from build123d import *

# Parameters (mm, degrees)
F0_W      = 44
F0_H      = 60
F1_DEPTH  = 20
F2_W      = 2.5
F2_H      = 17
F3_DEPTH  = 20
F4_T      = -1.5
F5_W      = 5
F5_H      = 15
F6_DEPTH  = 2
F7_W      = 14
F7_H      = 2
F7_H_2    = 14
F8_DEPTH  = 7
F10_DEPTH = 14
F11_W     = 4
F11_H     = 4
F12_DEPTH = 18.5
F13_R     = 1.05
F14_DEPTH = 15
F15_W     = 7.7
F15_H     = 4.2
F16_DEPTH = 1.5
F17_W     = 2
F17_H     = 43.7
F17_H_2   = 39.7
F18_DEPTH = 5
F19_W     = 3
F19_H     = 10
F20_DEPTH = 12
F21_W     = 6
F21_H     = 2
F22_DEPTH = 10


# Not quite as in the source:
# - a pattern or mirror of a feature is missing from the dataset's text; its kind, count and spacing are read off the source's solid


with BuildPart() as f1:
    # F0 (on Top) → F1 (new body)
    with BuildSketch(Plane.XY):
        Rectangle(F0_W, F0_H)
    extrude(amount=F1_DEPTH)

    # F2 (on face) → F3 (cut)
    with BuildSketch(Plane.XY.offset(20)):
        with Locations((20.75, 0)):
            Rectangle(F2_W, F2_H)
        with Locations((-20.75, 0)):
            Rectangle(F2_W, F2_H)
    extrude(amount=-F3_DEPTH, mode=Mode.SUBTRACT)

    # F4
    f4_openings = [f1.faces().sort_by_distance(p)[0] for p in [
        (0, 0, 20),
    ]]
    offset(amount=F4_T, openings=f4_openings, kind=Kind.INTERSECTION)

    # F5 (on face) → F6 (cut)
    with BuildSketch(Plane(origin=(0, 0, 0), x_dir=(1, 0, 0), z_dir=(0, 0, -1))):
        with Locations((-16.5, -21)):
            Rectangle(F5_W, F5_H)
    extrude(amount=-F6_DEPTH, mode=Mode.SUBTRACT)

    # F7 (on face) → F8 (join)
    with BuildSketch(Plane.YZ.offset(19.5)):
        with Locations((0, 21)):
            Rectangle(F7_W, F7_H)
        with Locations((0, 13)):
            Rectangle(F7_W, F7_H_2)
    f8 = extrude(amount=F8_DEPTH)

    # F8_copies: F8 across plane
    add(f8.mirror(Plane(origin=(0, 0, 0), x_dir=(0, 0, -1), z_dir=(-1, 0, 0))))

    # F9 (on face) → F10 (cut)
    with BuildSketch(Plane.XZ.offset(7)):
        Polygon((23, 16.5), (19.5, 6), (26.5, 6), (26.5, 20), (22, 20), (22, 16.5), align=None)
    f10 = extrude(amount=-F10_DEPTH, mode=Mode.SUBTRACT)

    # F10_copies: F10 across plane
    add(f10.mirror(Plane(origin=(0, 0, 0), x_dir=(0, 0, -1), z_dir=(-1, 0, 0))), mode=Mode.SUBTRACT)

    # F11 (on face) → F12 (join, through all)
    with BuildSketch(Plane.XY.offset(1.5)):
        with Locations((18.5, 26.5)):
            Rectangle(F11_W, F11_H)
        with Locations((18.5, -26.5)):
            Rectangle(F11_W, F11_H)
        with Locations((-18.5, -26.5)):
            Rectangle(F11_W, F11_H)
        with Locations((-10, 26.5)):
            Rectangle(F11_W, F11_H)
    extrude(amount=F12_DEPTH)

    # F13 (on face) → F14 (cut)
    with BuildSketch(Plane.XY.offset(20)):
        with Locations((-10, 26.5)):
            Circle(F13_R)
        with Locations((18.5, 26.5)):
            Circle(F13_R)
        with Locations((18.5, -26.5)):
            Circle(F13_R)
        with Locations((-18.5, -26.5)):
            Circle(F13_R)
    extrude(amount=-F14_DEPTH, mode=Mode.SUBTRACT)

    # F15 (on face) → F16 (cut, through all)
    with BuildSketch(Plane.XZ.offset(-28.5)):
        with Locations((1.25, 7.1)):
            Rectangle(F15_W, F15_H)
    extrude(amount=-F16_DEPTH, mode=Mode.SUBTRACT)

    # F17 (on face) → F18 (join)
    with BuildSketch(Plane.XY.offset(1.5)):
        with Locations((11.6, 6.65)):
            Rectangle(F17_W, F17_H)
        Polygon((12.6, -15.2), (10.6, -15.2), (-8, -15.2), (-10, -15.2), (-10, -17.2), (12.6, -17.2), align=None)
        with Locations((-9, 4.65)):
            Rectangle(F17_W, F17_H_2)
    extrude(amount=F18_DEPTH)

    # F19 (on face) → F20 (join)
    with BuildSketch(Plane.XY.offset(1.5)):
        with Locations((19, 17.5)):
            Rectangle(F19_W, F19_H)
        with Locations((19, -17.5)):
            Rectangle(F19_W, F19_H)
        with Locations((-19, -17.5)):
            Rectangle(F19_W, F19_H)
    extrude(amount=F20_DEPTH)

    # F21 (on face) → F22 (cut)
    with BuildSketch(Plane.XY.offset(1.5)):
        with Locations((1.6, -16.2)):
            Rectangle(F21_W, F21_H)
    extrude(amount=F22_DEPTH, mode=Mode.SUBTRACT)


solid = f1.part
Verification items for the finished model (mm, model axes). A direction names the side the tool comes from. Coordinates: 2 decimals unless noted, no trailing zeros. Loops run counter-clockwise (first coordinate to the right, second up) from the corner with the lowest first, then second, coordinate; pieces in that order, holes last. Notation, with made-up numbers: (1, -40) -> (8, -40) arc R25 ccw to (8, -28) -> close; hole circle Ø2 at (15.5, 4.5). An arc over 180 degrees is marked (long way). Answer as a JSON object with one key per item and string values. Group by question number.
Item 1: Scan lines: probe 1 along Y at (x, z) = (-10, 12.5); probe 2 along Y at (x, z) = (-3, 5.75); probe 3 along Y at (x, z) = (-20, 17.5). Record each from-to range of solid material in increasing order.
Item 2: Tool access check on faces 1 (the flat face through (1, 29, 9.2)), 2 (the flat face through (-22, 0, 18)), 3 (the flat face through (18, 24.5, 11)), 4 (the flat face through (-26.5, 0, 21)). Record the directions out of +Z, -Z, +X, -X, +Y, -Y that give a thin tool (end or side, any length) a straight path to the whole face; none if there is none.
Item 3: Sectioned sample at B-B on y = -26.5. Record the boundary of the cut face in (x, z).
Item 4: Mould release check, pull along X, two halves, no side actions. Record for faces 5 (the flat face through (-17.5, -18, 7)), 6 (the cylindrical face through (17.67, 25.86, 12.6)), 7 (the flat face through (-19.5, -0.1, 5.7)): +X half, -X half, draft (parallel to the pull), parting line (faces both ways), or undercut.
Item 5: Sectioned sample at C-C on z = 18.75. State how many separate pieces and enclosed holes the cut face has, plus the area to 3 significant figures.
Item 6: Sectioned sample at D-D on y = -14. Record the boundary of the cut face in (x, z), plus the area to 4 significant figures.
Item 7: Depth check by flat-ended pin: pin 1 (8 mm diameter, centred on y = -5.5, z = 9, fed in from -X); pin 2 (12 mm diameter, centred on x = 14, y = 22.5, fed in from +Z); pin 3 (10 mm diameter, centred on y = -21.5, z = 11.5, fed in from +X); pin 4 (4 mm diameter, centred on x = -20, y = 0, fed in from -Z). Enter the tip coordinate at first touch or a pass-through.
Item 8: Sectioned sample at A-A on x = 14. Record the boundary of the cut face in (y, z), plus the area to 4 significant figures.
Evaluation:
{
 "1": {"probe 1": "y = -30 to -28.5, 24.5 to 25.45, 27.55 to 30", "probe 2": "y = -30 to -28.5, -17.2 to -15.2, 28.5 to 30", "probe 3": "y = -30 to -24.5, -10 to -8.5, -7 to 7, 8.5 to 10, 28.5 to 30"},
 "2": {"face 1": "+Y", "face 2": "-X, +Y, -Y", "face 3": "+Z", "face 4": "+Z, -Z, -X, +Y, -Y"},
 "3": {"outline": "(-22, 0) -> (22, 0) -> (22, 20) -> (19.55, 20) -> (19.55, 5) -> (17.45, 5) -> (17.45, 20) -> (16.5, 20) -> (16.5, 1.5) -> (-16.5, 1.5) -> (-16.5, 20) -> (-17.45, 20) -> (-17.45, 5) -> (-19.55, 5) -> (-19.55, 20) -> (-22, 20) -> close"},
 "4": {"face 5": "undercut", "face 6": "undercut", "face 7": "-X half"},
 "5": {"separate pieces": "1", "enclosed holes": "5", "area": "438 mm²"},
 "6": {"outline": "(-22, 0) -> (22, 0) -> (22, 20) -> (20.5, 20) -> (20.5, 13.5) -> (17.5, 13.5) -> (17.5, 1.5) -> (12.6, 1.5) -> (12.6, 6.5) -> (10.6, 6.5) -> (10.6, 1.5) -> (-8, 1.5) -> (-8, 6.5) -> (-10, 6.5) -> (-10, 1.5) -> (-17.5, 1.5) -> (-17.5, 13.5) -> (-20.5, 13.5) -> (-20.5, 20) -> (-22, 20) -> close", "area": "213.5 mm²"},
 "7": {"pin 1": "stops at x = -22", "pin 2": "stops at z = 20", "pin 3": "stops at x = 22", "pin 4": "stops at z = 0"},
 "8": {"outline": "(-30, 0) -> (30, 0) -> (30, 20) -> (28.5, 20) -> (28.5, 1.5) -> (-28.5, 1.5) -> (-28.5, 20) -> (-30, 20) -> close", "area": "145.5 mm²"}
}
